Geometry: final body of the model. Coordinates: model frame, mm. Face numbers are marked on the shaded views. A direction names the side the tool comes from. Give positions to 0.01 mm unless a question says otherwise; leave off trailing zeros. Order: outer loops, then holes, each group sorted by start corner. A loop starts at its lowest first (then second) coordinate and runs counter-clockwise, first axis right, second up. Notation, with made-up numbers: (50, -25.75) -> (94, -25.75) arc R26 cw to (94, 13.25) -> close; hole circle Ø7 at (-31.75, 75.5). An arc over 180 degrees is marked (long way). Answer in a Markdown table with one row per item. Add a question column.
Q1. Line query: line 1 along Z through (x, y) = (-10, 1.5); line 2 along X through (y, z) = (0.2, -8.75); line 3 along Z through (x, y) = (-12.5, 0.75). Output: solid intervals per line, ascending. Write a range as from..to.
Q2. Cut plane A-A on x = -2. Return the cut outline in (y, z) (3 decimals).
Q3. Cut plane D-D on y = 0.9. Return the cut outline in (x, z), and give its area (3 significant figures).
Q4. Cut plane B-B on z = 0.5. Return the cut outline in (x, y) (1 decimal).
Q5. Pull-direction query (Z, two-part tool) for the marked faces 1, 2 and 3; classes: +Z half, -Z half, draft (parallel to the pull), parting line (faces both ways), or undercut.
Q6. Cut plane C-C on x = -14.5. Return the cut outline in (y, z) (3 decimals), and give its area (3 significant figures).
Q7. Set-up query: the marked faces 4 and 5. Return all of +Z, -Z, +X, -X, +Y, -Y with unobstructed straight access to the full face (end or side cutting, diameter ignored); none if empty.
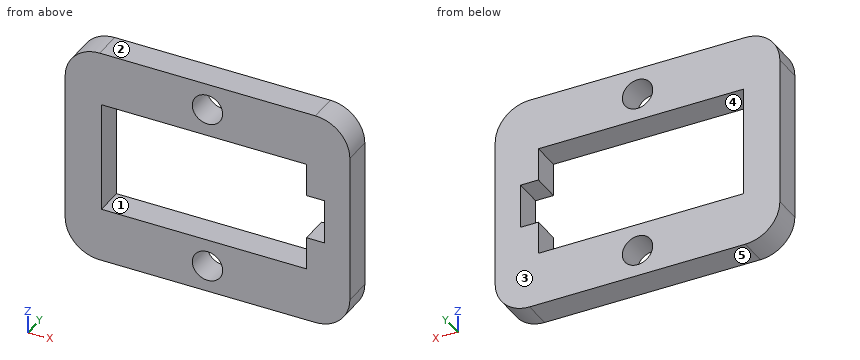
from build123d import *

# Parameters (mm, degrees)
SKETCH1_R           = 1.700000029
BOSS_EXTRUDE1_DEPTH = 3.175


with BuildPart() as part:
    # Sketch1 → Boss-Extrude1 (new body)
    with BuildSketch(Plane(origin=(0, 0, 0), x_dir=(1, 0, 0), z_dir=(0, 1, 0))):
        with BuildLine():
            Line((-1.425196706, 15.763070025), (-25.583614521, 15.763070025))
            ThreePointArc((-25.583614521, 15.763070025), (-28.310130326, 14.633710201), (-29.439490151, 11.907194396))
            Line((-29.439490151, 11.907194396), (-29.439490151, -4.88887146))
            ThreePointArc((-29.439490151, -4.88887146), (-28.308084251, -7.620326926), (-25.576628785, -8.751732825))
            Line((-25.576628785, -8.751732825), (-1.432182442, -8.751732825))
            ThreePointArc((-1.432182442, -8.751732825), (1.299273025, -7.620326926), (2.430678924, -4.88887146))
            Line((2.430678924, -4.88887146), (2.430678924, 11.907194396))
            ThreePointArc((2.430678924, 11.907194396), (1.301319099, 14.633710201), (-1.425196706, 15.763070025))
        make_face()
        with Locations(Location((-13.507869129, 12.77916147, 0), (0, 0, 270))):
            Circle(SKETCH1_R, mode=Mode.SUBTRACT)
        with Locations(Location((-13.507869129, -5.760838534, 0), (0, 0, 270))):
            Circle(SKETCH1_R, mode=Mode.SUBTRACT)
        Polygon((-2.416750389, 9.709339568), (-25.375916231, 9.709339568), (-25.375916231, -2.691010202), (-2.416750389, -2.691010202), (-2.416750389, 1.009089439), (-0.420102398, 1.009089439), (-0.420102398, 6.009239927), (-2.416750389, 6.009239927), align=None, mode=Mode.SUBTRACT)
    extrude(amount=BOSS_EXTRUDE1_DEPTH)


solid = part.part
Completed:
| question | item | result |
|---|---|---|
| 1 | line 1 | z = -15.76..-9.71, 2.69..8.75 |
| 1 | line 2 | x = -29.44..-25.38, -2.42..2.43 |
| 1 | line 3 | z = -15.76..-14.15, -11.41..-9.71, 2.69..4.39, 7.13..8.75 |
| 2 | outline | (0, -15.763) -> (3.175, -15.763) -> (3.175, -6.009) -> (0, -6.009) -> close; (0, -1.009) -> (3.175, -1.009) -> (3.175, 8.752) -> (0, 8.752) -> close |
| 3 | outline | (-29.44, -11.91) arc R3.86 ccw to (-25.58, -15.76) -> (-1.43, -15.76) arc R3.86 ccw to (2.43, -11.91) -> (2.43, 4.89) arc R3.86 ccw to (-1.43, 8.75) -> (-25.58, 8.75) arc R3.86 ccw to (-29.44, 4.89) -> close; hole (-25.38, -9.71) -> (-2.42, -9.71) -> (-2.42, -6.01) -> (-0.42, -6.01) -> (-0.42, -1.01) -> (-2.42, -1.01) -> (-2.42, 2.69) -> (-25.38, 2.69) -> close; hole circle Ø3.4 at (-13.51, -12.78); hole circle Ø3.4 at (-13.51, 5.76) |
| 3 | area | 456 mm² |
| 4 | outline | (-29.4, 0) -> (-25.4, 0) -> (-25.4, 3.2) -> (-29.4, 3.2) -> close; (-2.4, 0) -> (2.4, 0) -> (2.4, 3.2) -> (-2.4, 3.2) -> close |
| 5 | face 1 | undercut |
| 5 | face 2 | +Z half |
| 5 | face 3 | draft |
| 6 | outline | (0, -15.763) -> (3.175, -15.763) -> (3.175, -14.16) -> (0, -14.16) -> close; (0, -11.399) -> (3.175, -11.399) -> (3.175, -9.709) -> (0, -9.709) -> close; (0, 2.691) -> (3.175, 2.691) -> (3.175, 4.38) -> (0, 4.38) -> close; (0, 7.141) -> (3.175, 7.141) -> (3.175, 8.752) -> (0, 8.752) -> close |
| 6 | area | 20.9 mm² |
| 7 | face 4 | +Y, -Y |
| 7 | face 5 | -Z, +X, -X, +Y, -Y |
